Input: part model. Units: mm. Frame: model coordinates. A direction names the side the tool comes from. Give positions to 0.01 mm unless a question says otherwise; leave off trailing zeros. Loops run counter-clockwise (first coordinate to the right, second up) from the corner with the lowest first, then second, coordinate; pieces in that order, holes last. Notation, with made-up numbers: (65.5, 54) - (85.5, 54) arc R23 ccw to (85.5, 90) - close; hole circle Ø4 at (30, 61). An arc over 180 degrees is marked (long way). Answer as a JSON object with one key per item and string values. Group by question number.
(1) Section query B-B (y = -7.25). Return loops of the section in (x, z), plus the area to 3 significant figures.
(2) Section query D-D (y = -0.75). Return loops of the section in (x, z).
(3) Section query C-C (z = 0.75). Return loops of the section in (x, y).
(4) Material intervals for L1, parallel to Y at x = -10.25, z = 0.7; L2, parallel to Y at x = -8.25, z = 1; L3, parallel to Y at x = -2.75, z = 0.7, sorted ascending.
(5) Mould query, pull axis Y, two halves, no side actions, for faces 4 (the cylindrical face through (-13.354, -5.558, 0.751)), 5 (the cylindrical face through (-12.19, -7.28, 0.75)), 6 (the flat face through (-1, -2, 0)), 7 (the cylindrical face through (3.96, 5.853, 0.751)). Classes: +Y half, -Y half, draft (parallel to the pull), parting line (faces both ways), or undercut.
(6) Access query for faces 1 (the flat face through (-1, -2, 1.524)), 2 (the flat face through (-2.636, -3, 1)), 3 (the cylindrical face through (-11.17, 6.47, 0.75)). Directions: +Z, -Z, +X, -X, +Y, -Y. A direction counts if a zero-diameter tool reaches every point of the face in a straight line with its end or side. Return the directions, or none.
(7) Section query A-A (x = -6.5). Return loops of the section in (y, z).
```python
from build123d import *

# Parameters (mm, degrees)
BOSS_EXTRUDE1_DEPTH = 1.524


with BuildPart() as part:
    # Sketch1 → Boss-Extrude1 (new body)
    with BuildSketch(Plane.XY):
        with BuildLine():
            Line((-10.900934465, -3.68364082), (-2.635951713, -3.681036987))
            Line((-2.635951713, -3.681036987), (-2.635951713, -2.155055787))
            Line((-2.635951713, -2.155055787), (-10.901683213, -2.157042615))
            ThreePointArc((-10.901683213, -2.157042615), (-11.317544758, 0.15997729), (-9.511729503, 1.670127391))
            ThreePointArc((-9.511729503, 1.670127391), (-7.892680295, 2.86711895), (-7.885754316, 4.88058888))
            ThreePointArc((-7.885754316, 4.88058888), (-11.223059029, 6.479724486), (-14.907398818, 6.132625428))
            ThreePointArc((-14.907398818, 6.132625428), (-10.400280149, 8.822736649), (-5.152538869, 8.932411295))
            ThreePointArc((-5.152538869, 8.932411295), (4.07543143, 5.777326615), (10.640409761, -1.4345424))
            ThreePointArc((10.640409761, -1.4345424), (13.031939874, -7.001943531), (13.500316897, -13.04313502))
            ThreePointArc((13.500316897, -13.04313502), (9.547445937, -9.965660072), (4.697121946, -8.71250483))
            ThreePointArc((4.697121946, -8.71250483), (-2.219244662, -7.205435551), (-9.293116928, -6.945212506))
            ThreePointArc((-9.293116928, -6.945212506), (-12.232846335, -7.286099179), (-15.105972143, -7.995578426))
            ThreePointArc((-15.105972143, -7.995578426), (-13.323913323, -5.527094328), (-10.900934465, -3.68364082))
        make_face()
    extrude(amount=BOSS_EXTRUDE1_DEPTH)


solid = part.part
```
Recorded:
{
 "1": {"outline": "(-14.68, 0) - (-12.03, 0) - (-12.03, 1.52) - (-14.68, 1.52) - close; (-1.88, 0) - (13.09, 0) - (13.09, 1.52) - (-1.88, 1.52) - close", "area": "26.9 mm^2"},
 "2": {"outline": "(-11.46, 0) - (10.26, 0) - (10.26, 1.52) - (-11.46, 1.52) - close"},
 "3": {"outline": "(-15.11, -8) arc R23.38 cw to (-9.29, -6.95) arc R39.87 cw to (4.7, -8.71) arc R12.34 cw to (13.5, -13.04) arc R18.54 ccw to (10.64, -1.43) arc R19.6 ccw to (-5.15, 8.93) arc R10.26 ccw to (-14.91, 6.13) arc R6.93 cw to (-7.89, 4.88) arc R2.24 cw to (-9.51, 1.67) arc R2.34 ccw to (-10.9, -2.16) - (-2.64, -2.16) - (-2.64, -3.68) - (-10.9, -3.68) arc R10.35 ccw to start"},
 "4": {"L1": "y = -7.01 to -3.68, -2.16 to 1.41, 6.23 to 8.86", "L2": "y = -6.9 to -3.68, -2.16 to 2.35, 5.18 to 9.2", "L3": "y = -7.14 to -3.68, -2.16 to 8.59"},
 "5": {"face 4": "undercut", "face 5": "-Y half", "face 6": "draft", "face 7": "+Y half"},
 "6": {"face 1": "+Z, +X, -X, +Y, -Y", "face 2": "+Z, -Z, -X", "face 3": "+Z, -Z"},
 "7": {"outline": "(-6.9, 0) - (-3.68, 0) - (-3.68, 1.52) - (-6.9, 1.52) - close; (-2.16, 0) - (9.17, 0) - (9.17, 1.52) - (-2.16, 1.52) - close"}
}
